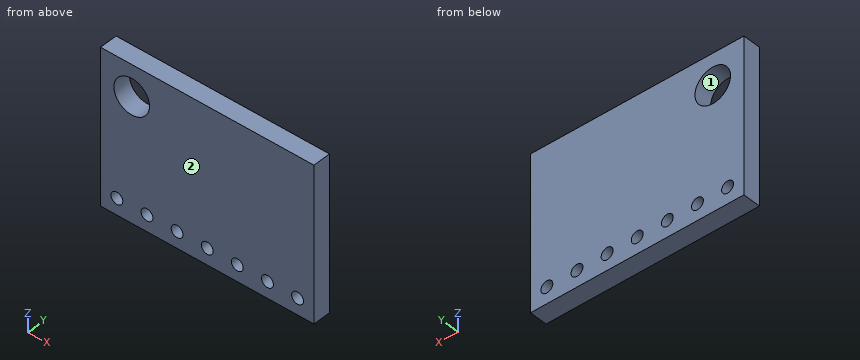
from build123d import *

# Parameters (mm, degrees)
SKETCH1_W           = 18
SKETCH1_H           = 13
SKETCH1_R           = 0.5
SKETCH1_R_2         = 1.5
BOSS_EXTRUDE1_DEPTH = 1.5


with BuildPart() as part:
    # Sketch1 → Boss-Extrude1 (new body)
    with BuildSketch(Plane(origin=(0, 0, 0), x_dir=(1, 0, 0), z_dir=(0, 1, 0))):
        with Locations((9, -6.5)):
            Rectangle(SKETCH1_W, SKETCH1_H)
        with Locations((1.38, -1.38)):
            Circle(SKETCH1_R, mode=Mode.SUBTRACT)
        with Locations((3.92, -1.38)):
            Circle(SKETCH1_R, mode=Mode.SUBTRACT)
        with Locations((6.46, -1.38)):
            Circle(SKETCH1_R, mode=Mode.SUBTRACT)
        with Locations((9, -1.38)):
            Circle(SKETCH1_R, mode=Mode.SUBTRACT)
        with Locations((11.54, -1.38)):
            Circle(SKETCH1_R, mode=Mode.SUBTRACT)
        with Locations((14.08, -1.38)):
            Circle(SKETCH1_R, mode=Mode.SUBTRACT)
        with Locations((16.62, -1.38)):
            Circle(SKETCH1_R, mode=Mode.SUBTRACT)
        with Locations((2.63, -10.37)):
            Circle(SKETCH1_R_2, mode=Mode.SUBTRACT)
    extrude(amount=-BOSS_EXTRUDE1_DEPTH)


solid = part.part
Geometry check sheet. Reference: the model listing, model coordinates, mm. Face numbers are marked on the shaded views. Coordinates: 2 decimals unless noted, no trailing zeros. Loops run counter-clockwise (first coordinate to the right, second up) from the corner with the lowest first, then second, coordinate; pieces in that order, holes last. Notation, with made-up numbers: (30, -24) - (82, -24) arc R32 ccw to (82, 10) - close; hole circle Ø4 at (-1.75, 46). An arc over 180 degrees is marked (long way). Use one line per item in the form item = value. Start each with the question number.
Item 1: Section check D-D, the plane z = 10.37. Enter the section's corners in (x, y).
Item 2: Section check A-A, the plane x = 14.08. Enter the section's corners in (y, z), and give its area (3 significant figures).
Item 3: Gauge pin test, flat end, axial feed: pin 1 (5 mm diameter, centred on x = 2.63, z = 10.37, fed in from -Y). Record the tip position at first contact, or that the pin passes through.
Item 4: Mould release check, pull along X, two halves, no side actions. Record for the marked faces 1 and 2: +X half, -X half, draft (parallel to the pull), parting line (faces both ways), or undercut.
Item 5: Thickness scan on probe 1 along Z at (x, y) = (2.63, -0.9); probe 2 along Z at (x, y) = (16.62, -1); probe 3 along X at (y, z) = (-0.3, 9.5). Record the ranges inside material, lowest first.
Item 6: Section check B-B, the plane y = -0.2. Give the number of separate pieces and of enclosed holes in the cut face, and give its area (3 significant figures).
Computed:
q1.outline = (0, -1.5) - (1.13, -1.5) - (1.13, 0) - (0, 0) - close; (4.13, -1.5) - (18, -1.5) - (18, 0) - (4.13, 0) - close
q2.outline = (-1.5, 0) - (0, 0) - (0, 0.88) - (-1.5, 0.88) - close; (-1.5, 1.88) - (0, 1.88) - (0, 13) - (-1.5, 13) - close
q2.area = 18.0 mm2
q3.pin_1 = -1.5
q4.face_1 = undercut
q4.face_2 = draft
q5.probe_1 = 0 to 8.87, 11.87 to 13
q5.probe_2 = 0 to 0.88, 1.88 to 13
q5.probe_3 = 0 to 1.41, 3.85 to 18
q6.separate_pieces = 1
q6.enclosed_holes = 8
q6.area = 221 mm2
